Drawing for the job (mm, zero at the part's lowest x, y, z). Round coordinates to 2 decimals unless told otherwise and drop trailing zeros. Loops run counter-clockwise (first coordinate to the right, second up) from the corner with the lowest first, then second, coordinate; pieces in that order, holes last. Notation, with made-up numbers: M 1,-33 L 55,-33 A22 ccw 55,-15 Z; hole C -25.75,37 d4. An arc over 180 degrees is marked long. Write each question's results on one line, items separated by ' | '.
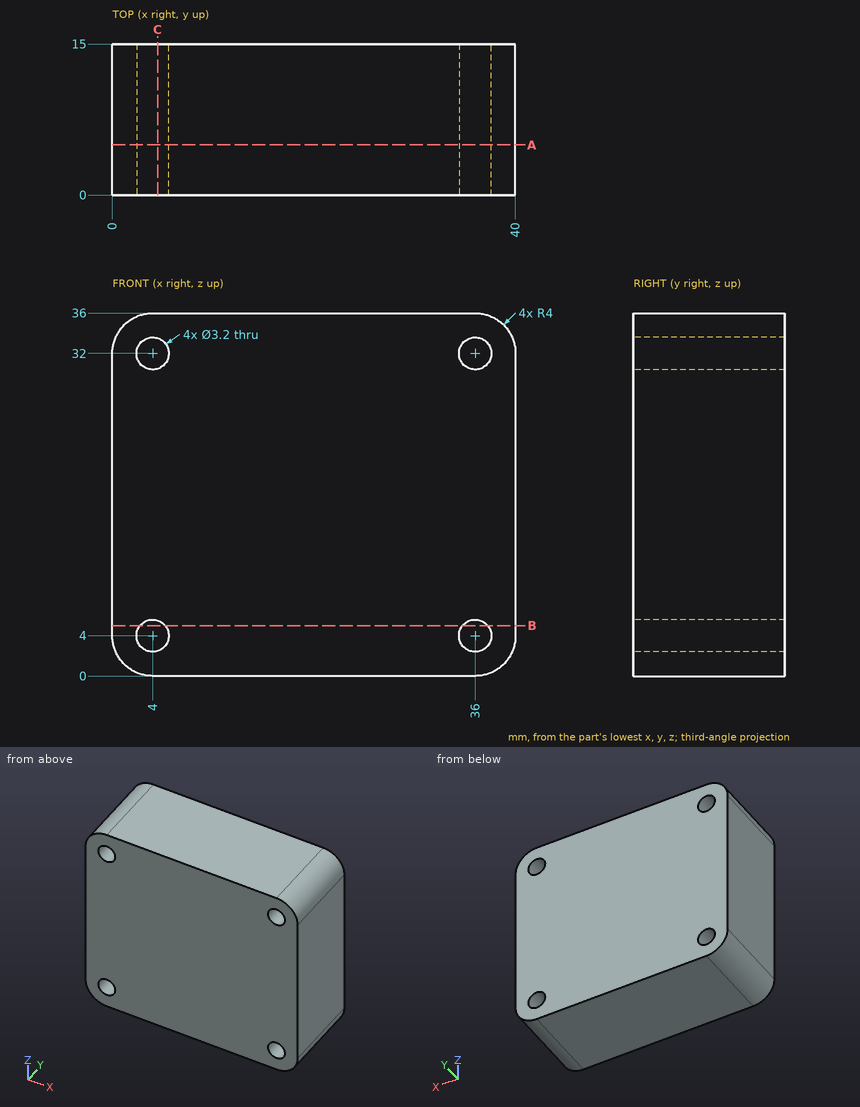
Item 1: Band-saw the part on B-B on z = 5. Give the cut face in (x, y), and give its area (3 significant figures).
Filled sheet:
outline: M 0,0 L 2.75,0 L 2.75,15 L 0,15 Z; M 5.25,0 L 34.75,0 L 34.75,15 L 5.25,15 Z; M 37.25,0 L 40,0 L 40,15 L 37.25,15 Z | area: 525 mm^2
Item 2: Band-saw the part on C-C on x = 4.5. Give the cut face in (y, z), and give its area (3 significant figures).
Filled sheet:
outline: M 0,0 L 15,0 L 15,2.48 L 0,2.48 Z; M 0,5.52 L 15,5.52 L 15,30.48 L 0,30.48 Z; M 0,33.52 L 15,33.52 L 15,36 L 0,36 Z | area: 449 mm^2
Item 3: Wall check: L1, parallel to X at y = 11.75, z = 4; L2, parallel to Z at x = 36, y = 9.25; L3, parallel to Z at x = 35, y = 4.25. Give the ranges that are in metal, low to high.
Filled sheet:
L1: 0 to 2.4, 5.6 to 34.4, 37.6 to 40 | L2: 0 to 2.4, 5.6 to 30.4, 33.6 to 36 | L3: 0 to 2.75, 5.25 to 30.75, 33.25 to 36
Item 4: Drop flat-ended pins along their axis: P1, Ø3, axis at x = 35.5, y = 9.5, coming from the -Z side; P2, Ø1.9, axis at x = 36, z = 32, coming from the +Y side. Give the stop position or say it passes through.
Filled sheet:
P1: z = 0 | P2: through
Item 5: Band-saw the part on A-A on y = 5. Give the cut face in (x, z), and give its area (3 significant figures).
Filled sheet:
outline: M 0,4 A4 ccw 4,0 L 36,0 A4 ccw 40,4 L 40,32 A4 ccw 36,36 L 4,36 A4 ccw 0,32 Z; hole C 4,4 d3.2; hole C 4,32 d3.2; hole C 36,4 d3.2; hole C 36,32 d3.2 | area: 1,390 mm^2
